Geometry check sheet. Reference: the model listing, model coordinates, mm. Coordinates: 2 decimals unless noted, no trailing zeros. Write each loop counter-clockwise with the first axis right and the second up, starting at its lowest first coordinate (ties: lowest second). Pieces come first, ordered by that corner, then holes. Notation, with made-up numbers: (69, 86) -> (90, 86) arc R6 cw to (90, 91) -> close; hole circle Ø4 at (84.25, -25.75). An arc over 180 degrees is marked (long way). Use a Markdown table: item, result.
```python
from build123d import *

# Parameters (mm, degrees)
CYLINDER001_W     = 10
CYLINDER001_H     = 10
CYLINDER001_ANGLE = 45
ARRAY_COUNT       = 6
CYLINDER_R        = 12
CYLINDER_DEPTH    = 10


with BuildPart() as array:
    # Cylinder001 → Cylinder001 (revolve)
    with BuildSketch(Plane(origin=(1, 1, 1), x_dir=(1, 0, 0), z_dir=(0, -1, 0))):
        with Locations((5, 5)):
            Rectangle(CYLINDER001_W, CYLINDER001_H)
    revolve(axis=Axis((1, 1, 1), (0, 0, 1)), revolution_arc=CYLINDER001_ANGLE)

    # Array: Array ×6 about axis
    array_axis = Axis((0, 0, 0), (0, 0, 1))


with BuildPart() as array_1:
    add(array.part)
    for i in range(1, ARRAY_COUNT):
        add(array.part.rotate(array_axis, i * 360 / ARRAY_COUNT))


with BuildPart() as cut:
    # Cylinder → Cylinder (new body)
    with BuildSketch(Plane.XY):
        Circle(CYLINDER_R)
    extrude(amount=CYLINDER_DEPTH)

    # Cut: cut Array
    add(array_1.part, mode=Mode.SUBTRACT)


solid = cut.part
```
Item 1: Section check C-C on x = 0. Record the boundary of the cut face in (y, z).
Answer block:
| item | result |
|---|---|
| outline | (-12, 0) -> (12, 0) -> (12, 10) -> (11.36, 10) -> (11.36, 1) -> (2, 1) -> (2, 10) -> (-2, 10) -> (-2, 1) -> (-11.36, 1) -> (-11.36, 10) -> (-12, 10) -> close |
Item 2: Section check A-A on z = 4.5. Record the boundary of the cut face in (x, y).
Answer block:
| item | result |
|---|---|
| outline | circle Ø24 at (0, 0); hole (-11.03, 2.95) -> (-1.37, 0.37) -> (-6.37, 9.03) arc R10 ccw to start; hole (-11, -1) arc R10 ccw to (-8.07, -8.07) -> (-1, -1) -> close; hole (-4.63, -10.03) arc R10 ccw to (2.95, -11.03) -> (0.37, -1.37) -> close; hole (-2.95, 11.03) -> (-0.37, 1.37) -> (4.63, 10.03) arc R10 ccw to start; hole (1, 1) -> (11, 1) arc R10 ccw to (8.07, 8.07) -> close; hole (1.37, -0.37) -> (6.37, -9.03) arc R10 ccw to (11.03, -2.95) -> close |
Item 3: Section check D-D on y = -2.5. Record the boundary of the cut face in (x, z).
Answer block:
| item | result |
|---|---|
| outline | (-11.74, 0) -> (11.74, 0) -> (11.74, 10) -> (9.33, 10) -> (9.33, 1) -> (2.6, 1) -> (2.6, 10) -> (0.67, 10) -> (0.67, 1) -> (-0.29, 1) -> (-0.29, 10) -> (-2.5, 10) -> (-2.5, 1) -> (-10.89, 1) -> (-10.89, 10) -> (-11.74, 10) -> close |
Item 4: Mould release check, pull along Y, two halves, no side actions. Record for faces 1 (the flat face through (7, 4, 1)), 2 (the cylindrical face through (-10.26, -4.78, 5.56)), 3 (the flat face through (0, 0, 10)): +Y half, -Y half, draft (parallel to the pull), parting line (faces both ways), or undercut.
Answer block:
| item | result |
|---|---|
| face 1 | undercut |
| face 2 | undercut |
| face 3 | draft |
Item 5: Thickness scan on L1, parallel to Y at x = 8.5, z = 5; L2, parallel to X at y = 4, z = 3.25; L3, parallel to X at y = -5, z = 8.5. Record the ranges inside material, lowest first. Write a range as [from, to].
Answer block:
| item | result |
|---|---|
| L1 | y = [-8.47, -7.37], [-2.28, 1], [7.61, 8.47] |
| L2 | x = [-11.31, -10.68], [-3.46, -1.07], [1.15, 4], [10.54, 11.31] |
| L3 | x = [-10.91, -10.17], [-5, -1.73], [1.34, 4.04], [10.23, 10.91] |
Item 6: Depth check by flat-ended pin: P1, Ø2.5, axis at x = -8, z = 5.5, coming from the -Y side; P2, Ø4, axis at y = -6, z = 4.5, coming from the -X side; P3, Ø1, axis at x = -2, z = 2, coming from the +Y side. Enter the tip coordinate at first touch or a pass-through.
Answer block:
| item | result |
|---|---|
| P1 | stops at y = -9.92 |
| P2 | stops at x = -11.31 |
| P3 | stops at y = 11.91 |
Item 7: Section check B-B on y = 5.75. Record the boundary of the cut face in (x, z).
Answer block:
| item | result |
|---|---|
| outline | (-10.53, 0) -> (10.53, 0) -> (10.53, 10) -> (9.8, 10) -> (9.8, 1) -> (5.75, 1) -> (5.75, 10) -> (2.17, 10) -> (2.17, 1) -> (-1.54, 1) -> (-1.54, 10) -> (-4.47, 10) -> (-4.47, 1) -> (-9.79, 1) -> (-9.79, 10) -> (-10.53, 10) -> close |
